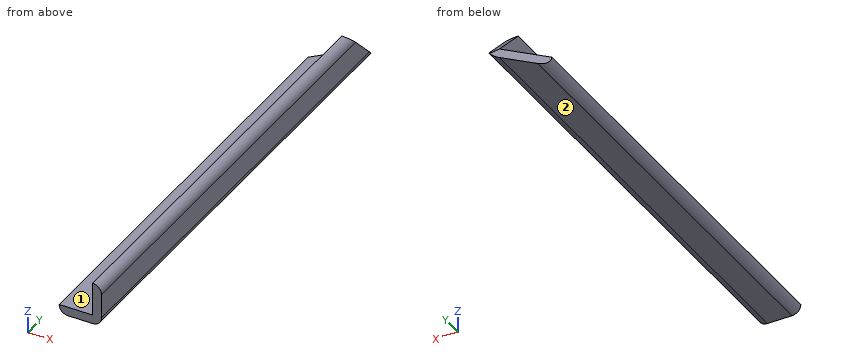
Autodesk Inventor part; units mm, degrees
ref_plane "YZ Plane" through (0, 0, 0) normal (1, 0, 0) x (0, 1, 0)
ref_plane "XZ Plane" through (0, 0, 0) normal (0, 1, 0) x (-1, 0, 0)
ref_plane "XY Plane" through (0, 0, 0) normal (0, 0, 1) x (1, 0, 0)
sketch "Skizze1" plane through (0, 0, 0) normal (0, 1, 0) x (-1, 0, 0)
  arc A0 (-4.6, 0) -> (0, -4.6) centre (0, 0) ccw
  line L0 (-4.6, 0) -> (-4.6, 12.6)
  arc A1 (0, 17.2) -> (-4.6, 12.6) centre (0, 12.6) ccw
  line L1 (0, 17.2) -> (0, 0)
  line L2 (0, 0) -> (17.2, 0)
  arc A2 (12.6, -4.6) -> (17.2, 0) centre (12.6, 0) ccw
  line L3 (12.6, -4.6) -> (0, -4.6)
  dimension "d0" = 4.6
  dimension "d1" = 21.8
extrude "Extrusion1" add sketch "Skizze1" along normal blind 248.6
sketch "Skizze2" plane through (4.6, 0, 12.6) normal (1, 0, 0) x (0, 0, -1)
  line L0 (17.2, 0) -> (17.2, 248.6)
  line L1 (17.2, 248.6) -> (-4.6, 226.8)
  line L2 (-4.6, 0) -> (-4.6, 248.6)
  line L3 (-4.6, 226.8) -> (-4.6, 248.6)
  line L4 (17.2, 248.6) -> (12.6, 248.6)
  line L5 (-4.6, 248.6) -> (17.2, 248.6)
  point P0 (12.6, 0)
  dimension "d4" = 45
extrude "Extrusion2" cut sketch "Skizze2" against normal through all
sketch "Skizze3" plane through (0, 0, -4.6) normal (0, 0, -1) x (-1, 0, 0)
  line L0 (-4.6, 0) -> (-4.6, 244)
  line L1 (17.2, 248.6) -> (-4.6, 248.6)
  line L2 (-4.6, 248.6) -> (17.2, 226.8)
  line L3 (17.2, 0) -> (17.2, 244)
  line L4 (17.2, 248.6) -> (17.2, 226.8)
  point P0 (0, 0)
  point P1 (0, 248.6)
  dimension "d9" = 45
extrude "Extrusion3" cut sketch "Skizze3" against normal through all
properties part number "eckeHochkant" material "Kiefer"
Could you check a few things on this model? Use its own coordinates, in mm. Face numbers are marked on the shaded views. A direction names the side the tool comes from. Give positions to 0.01 mm unless a question says otherwise; leave off trailing zeros. Order: outer loops, then holes, each group sorted by start corner. A loop starts at its lowest first (then second) coordinate and runs counter-clockwise, first axis right, second up. Notation, with made-up numbers: (83, 14.25) - (130, 14.25) arc R21 cw to (130, 28.25) - close; hole circle Ø4 at (57.25, 72). An arc over 180 degrees is marked (long way). One line per item, written item: value. Start each with the question number.
1. Imagine slicing it at A-A on y = 103. List the corners of the cut face in (x, z) for me.
2. For the marked faces 1 and 2, which set-ups out of +Z, -Z, +X, -X, +Y, -Y let a thin tool reach every point of the face, with its end or its side?
3. Imagine slicing it at B-B on z = 8. List the corners of the cut face in (x, y) for me, plus the area to 3 significant figures.
4. Imagine slicing it at C-C on x = -7.5. List the corners of the cut face in (y, z) for me, plus the area to 3 significant figures.
5. For P1, Ø8, axis at y = 91, z = 9.5, coming from the -X side; P2, Ø1, axis at x = -2, y = 145.5, coming from the +Z side, each with a flat end and sliding along its axis, tell me the tip position at first contact or that it passes through.
6. If I drill on probe 1 along Z at (x, y) = (-11.75, 145.5); probe 2 along X at (y, z) = (132, 2.5); probe 3 along X at (y, z) = (145.5, -0.5), over which ranges is the centre line in solid material (lowest first)?
Values:
1. outline: (-17.2, 0) arc R4.6 ccw to (-12.6, -4.6) - (0, -4.6) arc R4.6 ccw to (4.6, 0) - (4.6, 12.6) arc R4.6 ccw to (0, 17.2) - (0, 0) - close
2. face 1: +Z, -X, +Y, -Y
2. face 2: -Z, +X, -X, +Y, -Y
3. outline: (0, 0) - (4.6, 0) - (4.6, 236) - (0, 236) - close
3. area: 1,090 mm²
4. outline: (0, -4.6) - (236.5, -4.6) - (236.5, 0) - (0, 0) - close
4. area: 1,090 mm²
5. P1: x = 0
5. P2: z = 0
6. probe 1: -4.6 to 0
6. probe 2: 0 to 4.6
6. probe 3: -17.17 to 4.57
